Could you check a few things on this model? Use its own coordinates, in mm. Coordinates: 2 decimals unless noted, no trailing zeros. Write each loop counter-clockwise with the first axis right and the second up, starting at its lowest first coordinate (ties: lowest second). Pieces come first, ordered by that corner, then holes. Notation, with made-up numbers: M 84.25,36.5 L 128.25,36.5 A36 ccw 128.25,71.5 Z; hole C 60.25,73.25 d11. An arc over 180 degrees is marked long. Write item = value, one per line.
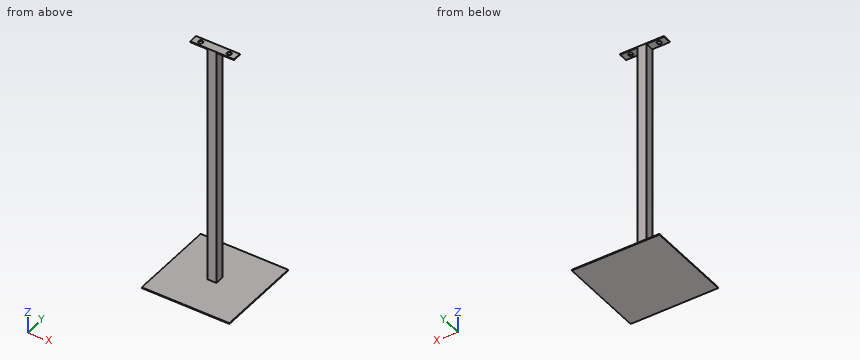
```python
from build123d import *

# Parameters (mm, degrees)
F0_W     = 400
F0_H     = 400
F1_DEPTH = 4
F2_W     = 40
F2_H     = 40
F3_DEPTH = 1100
F4_W     = 200
F4_H     = 40
F5_DEPTH = 4
F8_D     = 20
F8_DEPTH = 20
F9_D     = 20
F9_DEPTH = 20


with BuildPart() as f1:
    # F0 (on Top) → F1 (new body)
    with BuildSketch(Plane.XY):
        Rectangle(F0_W, F0_H)
    extrude(amount=F1_DEPTH)

    # F2 (on face) → F3 (join)
    with BuildSketch(Plane.XY.offset(4)):
        Rectangle(F2_W, F2_H)
    extrude(amount=F3_DEPTH)

    # F4 (on face) → F5 (join)
    with BuildSketch(Plane.XY.offset(1104)):
        Rectangle(F4_W, F4_H)
    extrude(amount=F5_DEPTH)

    # F8
    with Locations(Plane.XY.offset(1108)):
        with Locations((-65, 0)):
            Hole(F8_D / 2, depth=F8_DEPTH)

    # F9
    with Locations(Plane.XY.offset(1108)):
        with Locations((65, 0)):
            Hole(F9_D / 2, depth=F9_DEPTH)


solid = f1.part
```
Item 1: Imagine slicing it at C-C (y = 0). Write out the boundary of the cut face in (x, z).
Numbers:
outline = M -200,0 L 200,0 L 200,4 L 20,4 L 20,1104 L 55,1104 L 55,1108 L -55,1108 L -55,1104 L -20,1104 L -20,4 L -200,4 Z; M -100,1104 L -75,1104 L -75,1108 L -100,1108 Z; M 75,1104 L 100,1104 L 100,1108 L 75,1108 Z
Item 2: I'm going to push flat-ended pins straight in: P1, Ø2, axis at y = -8.5, z = 1106, coming from the -X side; P2, Ø10, axis at y = 28, z = 802.5, coming from the +X side; P3, Ø6, axis at x = 156, y = -56.5, coming from the -Z side; P4, Ø8, axis at x = 23, z = 381.5, coming from the -Y side. Where does each tip first touch, or does it pass through?
Numbers:
P1 = -100
P2 = through
P3 = 0
P4 = -20
Item 3: Imagine slicing it at A-A (x = -65). Write out the boundary of the cut face in (y, z).
Numbers:
outline = M -200,0 L 200,0 L 200,4 L -200,4 Z; M -20,1104 L -10,1104 L -10,1108 L -20,1108 Z; M 10,1104 L 20,1104 L 20,1108 L 10,1108 Z
Item 4: Imagine slicing it at B-B (x = 34.5). Write out the boundary of the cut face in (y, z), and give its area (3 significant figures).
Numbers:
outline = M -200,0 L 200,0 L 200,4 L -200,4 Z; M -20,1104 L 20,1104 L 20,1108 L -20,1108 Z
area = 1,760 mm²
Item 5: Imagine slicing it at D-D (y = 169.5). Write out the boundary of the cut face in (x, z), and give its area (3 significant figures).
Numbers:
outline = M -200,0 L 200,0 L 200,4 L -200,4 Z
area = 1,600 mm²
Item 6: If I drill on line 1 along Y through (x, z) = (-65, 1106.2); line 2 along Z through (x, y) = (24, -175.5); line 3 along Y through (x, z) = (-9, 821), over which ranges is the centre line in solid material (lowest first)?
Numbers:
line_1 = -20 to -10, 10 to 20
line_2 = 0 to 4
line_3 = -20 to 20
